The listing builds one solid part. Answer for the finished solid, in the listing's coordinates (mm). Give positions to 0.01 mm unless a question says otherwise; leave off trailing zeros. Write each loop counter-clockwise with the first axis right and the second up, starting at its lowest first coordinate (ties: lowest second). Pieces come first, ordered by that corner, then holes.
Autodesk Inventor part; units mm, degrees
ref_plane "YZ Plane" through (0, 0, 0) normal (1, 0, 0) x (0, 1, 0)
ref_plane "XZ Plane" through (0, 0, 0) normal (0, 1, 0) x (-1, 0, 0)
ref_plane "XY Plane" through (0, 0, 0) normal (0, 0, 1) x (1, 0, 0)
sketch "Skizze2" plane through (0, 0, 0) normal (0, 1, 0) x (-1, 0, 0)
  line L0 (0, 0) -> (52, 0)
  line L1 (52, 0) -> (52, 35)
  line L2 (52, 35) -> (0, 35)
  line L3 (0, 35) -> (0, 0)
  dimension "d3" = 52
  dimension "d4" = 35
extrude "Extrusion1" add sketch "Skizze2" along normal blind 2
sketch "Skizze3" plane through (0, 0, 0) normal (0, -1, 0) x (1, 0, 0)
  line L0 (0, 35) -> (0, 0)
  line L1 (-52, 0) -> (-52, 35)
  line L2 (-52, 17.5) -> (0, 17.5)
  line L3 (-33.5, 17.5) -> (-18.5, 17.5)
  line L4 (-33.5, 17.5) -> (-52, 17.5)
  line L5 (-18.5, 17.5) -> (0, 17.5)
  circle A0 centre (-33.5, 17.5) radius 1.525
  circle A1 centre (-18.5, 17.5) radius 1.525
  dimension "d7" = 15
  dimension "d8" = 3.05
  dimension "d9" = 3.05
extrude "Extrusion2" cut sketch "Skizze3" against normal through all
sketch "Skizze6" plane through (0, 0, 0) normal (0, -1, 0) x (1, 0, 0)
  line L0 (0, 0) -> (-52, 0)
  line L1 (0, 35) -> (0, 0)
  line L2 (-52, 35) -> (0, 35)
  line L3 (-52, 0) -> (-52, 35)
  line L4 (-47, 30) -> (-5, 30)
  line L5 (-5, 30) -> (-5, 5)
  line L6 (-5, 5) -> (-47, 5)
  line L7 (-47, 5) -> (-47, 30)
  dimension "d17" = 5
  dimension "d18" = 5
  dimension "d19" = 5
  dimension "d20" = 5
hole "Bohrung1" at (-5, 0, 5) at (-5, 0, 30) at (-47, 0, 30) at (-47, 0, 5) direction (0, 1, 0) diameter 4.1 end through all
fillet "Rundung2" radius 2 4 edges at (-52, 1, 35) (-52, 1, 0) (0, 1, 0) (0, 1, 35)
properties part number "frontcncld"
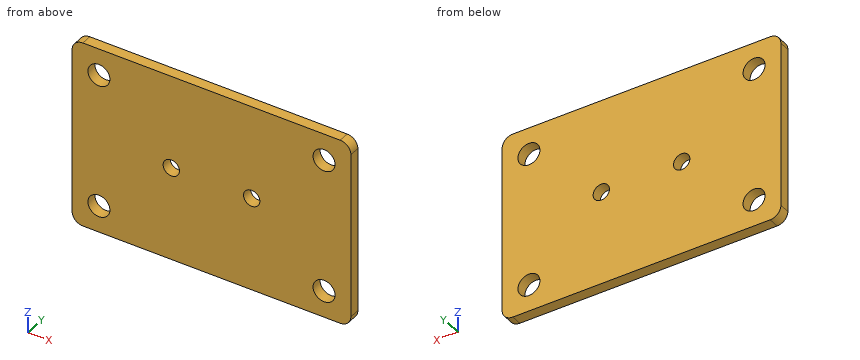
Item 1: A cutting plane is placed at A-A, the plane y = 1.2. Give the vertices of the cut face in (x, z) (3 decimals).
Conclusion:
outline: (-52, 2) arc R2 ccw to (-50, 0) - (-2, 0) arc R2 ccw to (0, 2) - (0, 33) arc R2 ccw to (-2, 35) - (-50, 35) arc R2 ccw to (-52, 33) - close; hole circle Ø4.1 at (-47, 5); hole circle Ø4.1 at (-47, 30); hole circle Ø3.05 at (-33.5, 17.5); hole circle Ø3.05 at (-18.5, 17.5); hole circle Ø4.1 at (-5, 5); hole circle Ø4.1 at (-5, 30)
Item 2: A cutting plane is placed at C-C, the plane z = 30. Give the vertices of the cut face in (x, y), plus the area to 3 significant figures.
Conclusion:
outline: (-52, 0) - (-49.05, 0) - (-49.05, 2) - (-52, 2) - close; (-44.95, 0) - (-7.05, 0) - (-7.05, 2) - (-44.95, 2) - close; (-2.95, 0) - (0, 0) - (0, 2) - (-2.95, 2) - close
area: 87.6 mm2
Item 3: A cutting plane is placed at B-B, the plane x = -18.5. Give the vertices of the cut face in (y, z) (3 decimals).
Conclusion:
outline: (0, 0) - (2, 0) - (2, 15.975) - (0, 15.975) - close; (0, 19.025) - (2, 19.025) - (2, 35) - (0, 35) - close
Item 4: Consider probe 1 along Z at (x, y) = (-5, 1.55); probe 2 along X at (y, z) = (1.7, 17.5) (3 decimals); probe 3 along X at (y, z) = (0.75, 5). Determine where each line is inside the solid, lowest interval first.
Conclusion:
probe 1: z = 0 to 2.95, 7.05 to 27.95, 32.05 to 35
probe 2: x = -52 to -35.025, -31.975 to -20.025, -16.975 to 0
probe 3: x = -52 to -49.05, -44.95 to -7.05, -2.95 to 0
Item 5: A cutting plane is placed at D-D, the plane x = -5. Give the vertices of the cut face in (y, z), plus the area to 3 significant figures.
Conclusion:
outline: (0, 0) - (2, 0) - (2, 2.95) - (0, 2.95) - close; (0, 7.05) - (2, 7.05) - (2, 27.95) - (0, 27.95) - close; (0, 32.05) - (2, 32.05) - (2, 35) - (0, 35) - close
area: 53.6 mm2
Item 6: This flat-tipped pin is pushed along its axis until it touches: P1, Ø4, axis at x = -33.5, z = 17.5, coming from the +Y side. Where does it stop, or does it pass through?
Conclusion:
P1: stops at y = 2
